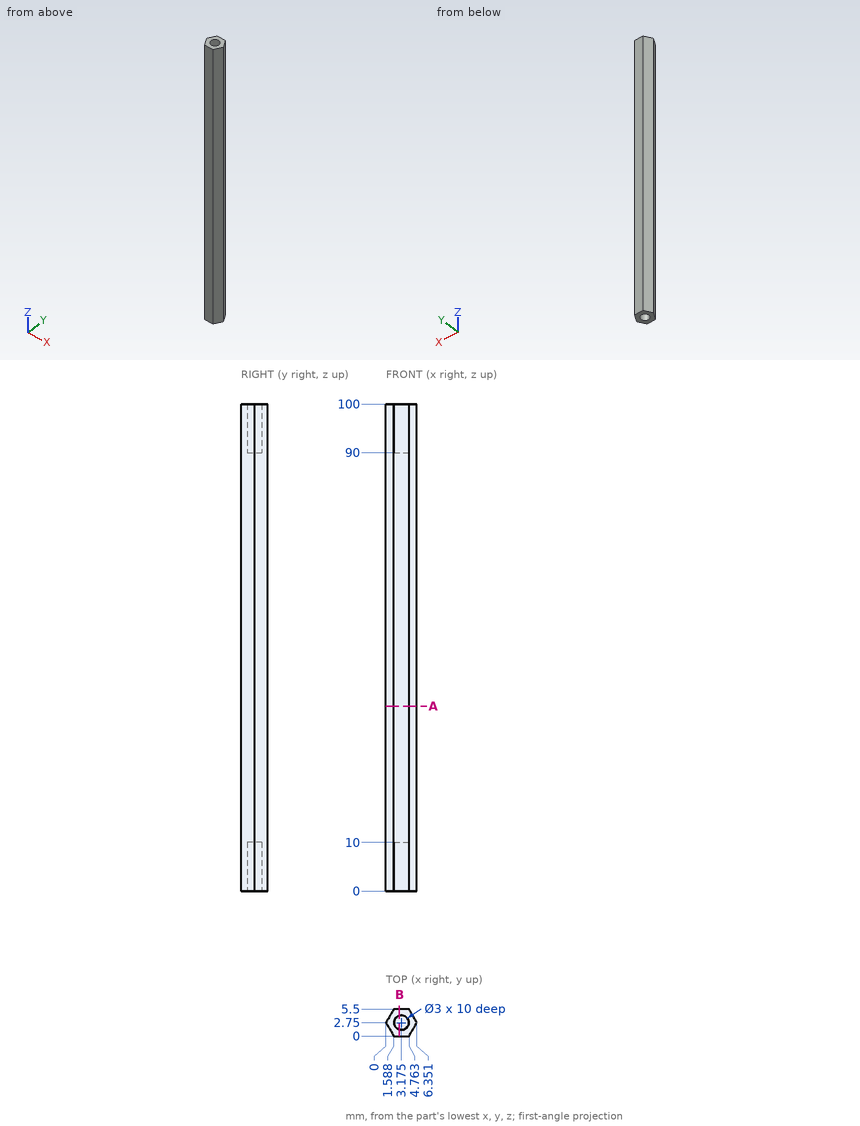
Check sheet for the drawn part. Datum: minimum x, y, z corner. Units: mm. Give positions to 0.01 mm unless a question says otherwise; leave off trailing zeros. Write each loop counter-clockwise with the first axis right and the second up, starting at its lowest first coordinate (ties: lowest second). Pieces come first, ordered by that corner, then holes.
(1) Material ranges on line 1 (Z direction, x = 3.5, y = 2.05); line 2 (X direction, y = 1.7, z = 95) (1 decimal); line 3 (X direction, y = 4.25, z = 21.5) (1 decimal), recorded low to high.
(2) Gauge pin test, flat ends, axial feed: pin 1 (2 mm diameter, centred on y = 1.5, z = 77.5, fed in from -X) (1 decimal); pin 2 (2.5 mm diameter, centred on x = 3.18, y = 2.75, fed in from +Z). Record the tip position at first contact, or that the pin passes through.
(3) Cross-section at B-B (x = 2.75). Enter the section's corners in (y, z).
(4) Cross-section at A-A (z = 38). Enter the section's corners in (x, y), plus the area to 3 significant figures.
Worked out:
1. line 1: z = 10 to 90
1. line 2: x = 0.6 to 2.1, 4.2 to 5.7
1. line 3: x = 0.9 to 5.5
2. pin 1: stops at x = 0.1
2. pin 2: stops at z = 90
3. outline: (0, 0) - (1.31, 0) - (1.31, 10) - (4.19, 10) - (4.19, 0) - (5.5, 0) - (5.5, 100) - (4.19, 100) - (4.19, 90) - (1.31, 90) - (1.31, 100) - (0, 100) - close
4. outline: (0, 2.75) - (1.59, 0) - (4.76, 0) - (6.35, 2.75) - (4.76, 5.5) - (1.59, 5.5) - close
4. area: 26.2 mm2
